Model file for the job. Use its own axes, mm. Give positions to 0.01 mm unless a question says otherwise; leave off trailing zeros. Loops run counter-clockwise (first coordinate to the right, second up) from the corner with the lowest first, then second, coordinate; pieces in that order, holes last. Notation, with made-up numbers: (6, 78) - (29, 78) arc R22 cw to (29, 102) - close; hole circle Ø6 at (67.5, 60). An arc over 180 degrees is marked (long way). Use a Markdown table: item, result.
Autodesk Inventor part; units mm, degrees
ref_plane "YZ Plane" through (0, 0, 0) normal (1, 0, 0) x (0, 1, 0)
ref_plane "XZ Plane" through (0, 0, 0) normal (0, 1, 0) x (-1, 0, 0)
ref_plane "XY Plane" through (0, 0, 0) normal (0, 0, 1) x (1, 0, 0)
sketch "Sketch1" plane through (0, 0, 0) normal (0, 0, 1) x (1, 0, 0)
  point P0 (0, 0)
sketch "Sketch2" plane through (0, 0, 0) normal (0, 0, 1) x (1, 0, 0)
  line L0 (94.9998, -95.0001) -> (-94.9998, -95.0001)
  line L1 (-94.9998, -95.0001) -> (-94.9998, 95.0001)
  line L2 (-94.9998, 95.0001) -> (94.9998, 95.0001)
  line L3 (94.9998, 95.0001) -> (94.9998, -95.0001)
  line L4 (94.9998, -95.0001) -> (-94.9998, 95.0001) construction
  line L5 (-94.9998, -95.0001) -> (94.9998, 95.0001) construction
  point P0 (0, 0)
extrude "Extrusion1" add sketch "Sketch2" along normal blind 3
sketch "Sketch3" plane through (0, 0, 3) normal (0, 0, 1) x (1, 0, 0)
  circle A0 centre (70, 80) radius 1.5001
  circle A1 centre (70, -80) radius 1.5001
  circle A2 centre (-70, 80) radius 1.5001
  circle A3 centre (-70, -80) radius 1.5001
extrude "Extrusion2" cut sketch "Sketch3" against normal blind 3
fillet "Fillet1" radius 25 1 edges at (94.9998, 95.0001, 1.5)
fillet "Fillet2" radius 25 1 edges at (94.9998, -95.0001, 1.5)
fillet "Fillet3" radius 25 1 edges at (-94.9998, -95.0001, 1.5)
fillet "Fillet4" radius 25 1 edges at (-94.9998, 95.0001, 1.5)
sketch "Pi mount holes" plane through (0, 0, 3) normal (0, 0, 1) x (1, 0, 0)
  circle A0 centre (24, -30.5) radius 1.2502
  circle A1 centre (-34, -30.5) radius 1.2502
  circle A2 centre (-34, -79.5) radius 1.2502
  circle A3 centre (24, -79.5) radius 1.2502
sketch "B205 mount holes" plane through (0, 0, 3) normal (0, 0, 1) x (1, 0, 0)
  circle A0 centre (20.32, 30.48) radius 1.5002
  circle A1 centre (-45.72, 30.48) radius 1.5002
  circle A2 centre (-45.72, -12.7) radius 1.5002
  circle A3 centre (20.32, -12.7) radius 1.5002
sketch "RM3100 mount holes" plane through (0, 0, 3) normal (0, 0, 1) x (1, 0, 0)
  circle A0 centre (0, 9) radius 0.9999
  circle A1 centre (0, -9) radius 0.9999
sketch "Pololu mount holes" plane through (0, 0, 3) normal (0, 0, 1) x (1, 0, 0)
  circle A0 centre (-73.2965, -23.9932) radius 1.1973
  circle A1 centre (-88.2965, -23.9932) radius 1.1973
  circle A2 centre (-73.2965, -59.4932) radius 1.1973
  circle A3 centre (-88.2965, -59.4932) radius 1.1973
sketch "B205 cable cutout" plane through (0, 0, 3) normal (0, 0, 1) x (1, 0, 0)
  line L0 (-76.0426, -14.5593) -> (-76.0426, 37.4411) construction
  line L1 (-81.5424, -9.0595) -> (-81.5424, 31.9413)
  line L2 (-70.5428, 31.9413) -> (-70.5428, -9.0595)
  arc A0 (-81.5424, -9.0595) -> (-70.5428, -9.0595) centre (-76.0426, -9.0595) ccw
  arc A1 (-70.5428, 31.9413) -> (-81.5424, 31.9413) centre (-76.0426, 31.9413) ccw
  point P0 (0, 0)
  point P1 (-76.0426, 11.4409)
sketch "Pi cable cutout" plane through (0, 0, 3) normal (0, 0, 1) x (1, 0, 0)
  line L0 (65.7382, -60.7056) -> (65.7382, 5.2939) construction
  line L1 (60.7378, -55.7052) -> (60.7378, 0.2935)
  line L2 (70.7387, 0.2935) -> (70.7387, -55.7052)
  arc A0 (60.7378, -55.7052) -> (70.7387, -55.7052) centre (65.7382, -55.7052) ccw
  arc A1 (70.7387, 0.2935) -> (60.7378, 0.2935) centre (65.7382, 0.2935) ccw
  point P0 (0, 0)
  point P1 (65.7382, -27.7058)
sketch "Imperial standoffs" plane through (0, 0, 3) normal (0, 0, 1) x (1, 0, 0)
  circle A0 centre (80, 80) radius 1.4302
  circle A1 centre (-80, -80) radius 1.4302
  circle A2 centre (80, -80) radius 1.4302
  circle A3 centre (-80, 80) radius 1.4302
extrude "Extrusion3" cut sketch "B205 cable cutout" against normal blind 10
extrude "Extrusion4" cut sketch "Pi cable cutout" against normal blind 10
extrude "Extrusion5" cut sketch "Imperial standoffs" against normal blind 10
extrude "Extrusion6" cut sketch "Pololu mount holes" against normal blind 10
extrude "Extrusion7" cut sketch "B205 mount holes" against normal blind 10
extrude "Extrusion8" cut sketch "RM3100 mount holes" against normal blind 10
extrude "Extrusion9" cut sketch "Pi mount holes" against normal blind 10
properties part number "payload_bay_square_drill_holes"
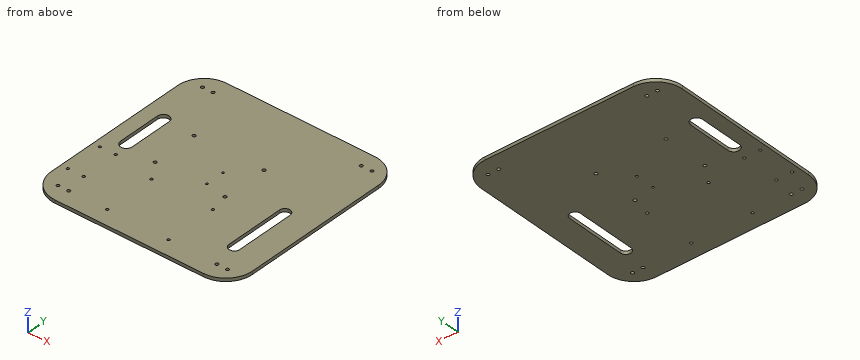
(1) Slice it at C-C, the plane z = 2.25. Count the separate pieces of the cut face and the enclosed holes in it, plus the area to 3 significant figures.
Computed:
| item | result |
|---|---|
| separate pieces | 1 |
| enclosed holes | 24 |
| area | 34,300 mm² |
(2) Slice it at A-A, the plane y = 26.5. Write the cut outline in (x, z), plus the area to 3 significant figures.
Computed:
| item | result |
|---|---|
| outline | (-95, 0) - (-81.54, 0) - (-81.54, 3) - (-95, 3) - close; (-70.54, 0) - (95, 0) - (95, 3) - (-70.54, 3) - close |
| area | 537 mm² |
(3) Pin check, flat tip, straight feed: P1, Ø3.5, axis at x = -34, y = -30.5, coming from the -Z side. Stop position of the tip, or through.
Computed:
| item | result |
|---|---|
| P1 | z = 0 |
(4) Drill centre lines: probe 1 along Y at (x, z) = (0, 2); probe 2 along Y at (x, z) = (-70, 1.3); probe 3 along X at (y, z) = (0, 1.7). Where is each one in solid material? Low to high. Write a range as [from, to].
Computed:
| item | result |
|---|---|
| probe 1 | [-95, -10], [-8, 8], [10, 95] |
| probe 2 | [-95, -81.5], [-78.5, 78.5], [81.5, 95] |
| probe 3 | [-95, -81.54], [-70.54, 60.74], [70.74, 95] |
(5) Slice it at B-B, the plane y = -52. Write the cut outline in (x, z), plus the area to 3 significant figures.
Computed:
| item | result |
|---|---|
| outline | (-95, 0) - (60.74, 0) - (60.74, 3) - (-95, 3) - close; (70.74, 0) - (95, 0) - (95, 3) - (70.74, 3) - close |
| area | 540 mm² |
